Can you work these out from the model? Positions are in its coordinate system, mm. Coordinates: 2 decimals unless noted, no trailing zeros. Write each loop counter-clockwise with the first axis right and the second up, starting at its lowest first coordinate (ties: lowest second). Pieces come first, ordered by that corner, then holes. Notation, with made-up numbers: (-2, 40) - (36, 40) arc R28 cw to (36, 73) - close; hole circle Ø7 at (49, 61.5). An arc over 180 degrees is marked (long way). One line per question, with ' | ' between items. Start each with the question number.
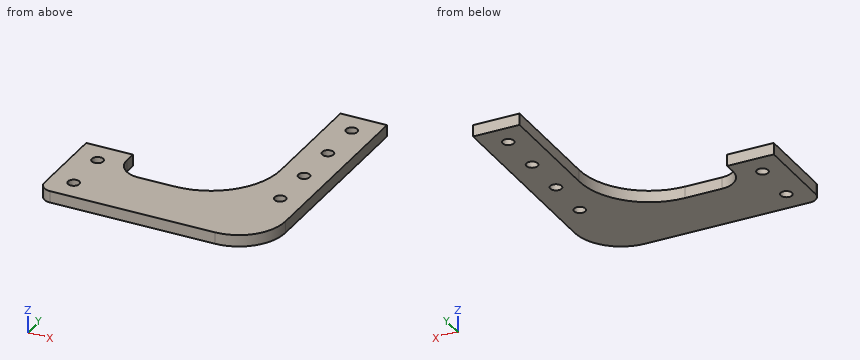
Autodesk Inventor part; units mm, degrees
ref_plane "YZ Plane" through (0, 0, 0) normal (1, 0, 0) x (0, 1, 0)
ref_plane "XZ Plane" through (0, 0, 0) normal (0, 1, 0) x (-1, 0, 0)
ref_plane "XY Plane" through (0, 0, 0) normal (0, 0, 1) x (1, 0, 0)
sketch "Sketch1" plane through (0, 0, 0) normal (0, 0, 1) x (1, 0, 0)
  line L0 (0, 0) -> (0, 133.35)
  line L1 (0, 133.35) -> (-25.4, 133.35)
  line L2 (-25.4, 133.35) -> (-25.4, 69.85)
  line L3 (-63.5, 31.75) -> (-83.693, 31.75)
  line L4 (-96.393, 44.45) -> (-96.393, 50.8)
  line L5 (-96.393, 50.8) -> (-121.793, 50.8)
  line L6 (-121.793, 50.8) -> (-121.793, 0)
  line L7 (-121.793, 0) -> (0, 0)
  arc A0 (-96.393, 44.45) -> (-83.693, 31.75) centre (-83.693, 44.45) ccw
  arc A1 (-63.5, 31.75) -> (-25.4, 69.85) centre (-63.5, 69.85) ccw
  circle A2 centre (-12.7, 120.65) radius 3.1
  circle A3 centre (-12.7, 95.25) radius 3.1
  circle A4 centre (-12.7, 69.85) radius 3.1
  circle A5 centre (-12.7, 44.45) radius 3.1
  circle A6 centre (-109.093, 38.1) radius 3.1
  circle A7 centre (-109.093, 12.7) radius 3.1
  point P0 (-25.4, 31.75)
  point P1 (-96.393, 31.75)
  dimension "d0" = 133.35
  dimension "d1" = 25.4
  dimension "d2" = 101.6
  dimension "d3" = 70.993
  dimension "d4" = 19.05
  dimension "d5" = 25.4
  dimension "d6" = 12.7
  dimension "d7" = 38.1
  dimension "d8" = 6.2
  dimension "d9" = 12.7
  dimension "d10" = 12.7
  dimension "d13" = 25.4
  dimension "d18" = 6.2
  dimension "d19" = 12.7
  dimension "d20" = 12.7
  dimension "d21" = 6.2
  dimension "d22" = 25.4
extrude "Extrusion1" add sketch "Sketch1" along normal blind 6.35
fillet "Fillet1" radius 25.4 1 edges at (0, 0, 3.175)
fillet "Fillet2" radius 6.35 1 edges at (-121.793, 0, 3.175)
properties part number "sidethrustalum" material "Aluminum 6061"
(1) If I drill on probe 1 along X at (y, z) = (45.5, 1); probe 2 along X at (y, z) = (106, 1); probe 3 along Y at (x, z) = (-81.5, 5), over which ranges is the centre line in solid material (lowest first)?
(2) If we section it at C-C on x = -12.7: List the corners of the cut face in (y, z) for me.
(3) I'm going to push flat-ended pins straight in: pin 1 (3 mm diameter, centred on x = -79.5, z = 5.5, fed in from +Y); pin 2 (3.5 mm diameter, centred on x = -12.7, y = 95.25, fed in from -Z); pin 3 (3 mm diameter, centred on x = -86, z = 5.5, fed in from +Y). Where does each tip first touch, or does it pass through?
(4) If we section it at B-B on z = 2.25: List the corners of the cut face in (x, y) for me.
(5) If we section it at A-A on y = 95.25: List the corners of the cut face in (x, z) for me, plus the area to 3 significant figures.
(6) If we section it at D-D on y = 38.1: List the corners of the cut face in (x, z) for me, plus the area to 3 significant figures.
Values:
1) probe 1: -121.79 to -96.39, -34.2 to -15.62, -9.78 to 0 | probe 2: -25.4 to 0 | probe 3: 0 to 31.75
2) outline: (3.4, 0) - (41.35, 0) - (41.35, 6.35) - (3.4, 6.35) - close; (47.55, 0) - (66.75, 0) - (66.75, 6.35) - (47.55, 6.35) - close; (72.95, 0) - (92.15, 0) - (92.15, 6.35) - (72.95, 6.35) - close; (98.35, 0) - (117.55, 0) - (117.55, 6.35) - (98.35, 6.35) - close; (123.75, 0) - (133.35, 0) - (133.35, 6.35) - (123.75, 6.35) - close
3) pin 1: y = 31.75 | pin 2: through | pin 3: y = 32.33
4) outline: (-121.79, 6.35) arc R6.35 ccw to (-115.44, 0) - (-25.4, 0) arc R25.4 ccw to (0, 25.4) - (0, 133.35) - (-25.4, 133.35) - (-25.4, 69.85) arc R38.1 cw to (-63.5, 31.75) - (-83.69, 31.75) arc R12.7 cw to (-96.39, 44.45) - (-96.39, 50.8) - (-121.79, 50.8) - close; hole circle Ø6.2 at (-109.09, 12.7); hole circle Ø6.2 at (-109.09, 38.1); hole circle Ø6.2 at (-12.7, 44.45); hole circle Ø6.2 at (-12.7, 69.85); hole circle Ø6.2 at (-12.7, 95.25); hole circle Ø6.2 at (-12.7, 120.65)
5) outline: (-25.4, 0) - (-15.8, 0) - (-15.8, 6.35) - (-25.4, 6.35) - close; (-9.6, 0) - (0, 0) - (0, 6.35) - (-9.6, 6.35) - close | area: 122 mm2
6) outline: (-121.79, 0) - (-112.19, 0) - (-112.19, 6.35) - (-121.79, 6.35) - close; (-105.99, 0) - (-94.69, 0) - (-94.69, 6.35) - (-105.99, 6.35) - close; (-42.44, 0) - (0, 0) - (0, 6.35) - (-42.44, 6.35) - close | area: 402 mm2
